Drawing for the job (mm, zero at the part's lowest x, y, z). Give positions to 0.01 mm unless a question says otherwise; leave off trailing zeros. Write each loop counter-clockwise with the first axis right and the second up, starting at its lowest first coordinate (ties: lowest second). Pieces come first, ordered by that corner, then holes. Notation, with made-up numbers: M 26.25,20.5 L 56.25,20.5 A30 cw 56.25,44.5 Z; hole C 74.5,67.5 d8. An arc over 180 degrees is marked long. Use CSV: the item, a comma, the result in double quotes. Start each with the question number.
1. Drill centre lines: line 1 along X through (y, z) = (14, 5); line 2 along X through (y, z) = (30.5, 7.25). Where is each one in solid material? Low to high. Write a range as from..to.
2. Drop flat-ended pins along their axis: pin 1 Ø1 at (y, z) = (12.5, 7) entering from +X; pin 2 Ø4 at (y, z) = (14.5, 7) entering from +X; pin 3 Ø3 at (x, y) = (68, 27.5) entering from -Z. Give the stop position or say it passes through.
3. Band-saw the part on A-A, the plane z = 7.75. List the corners of the cut face in (x, y) (3 decimals).
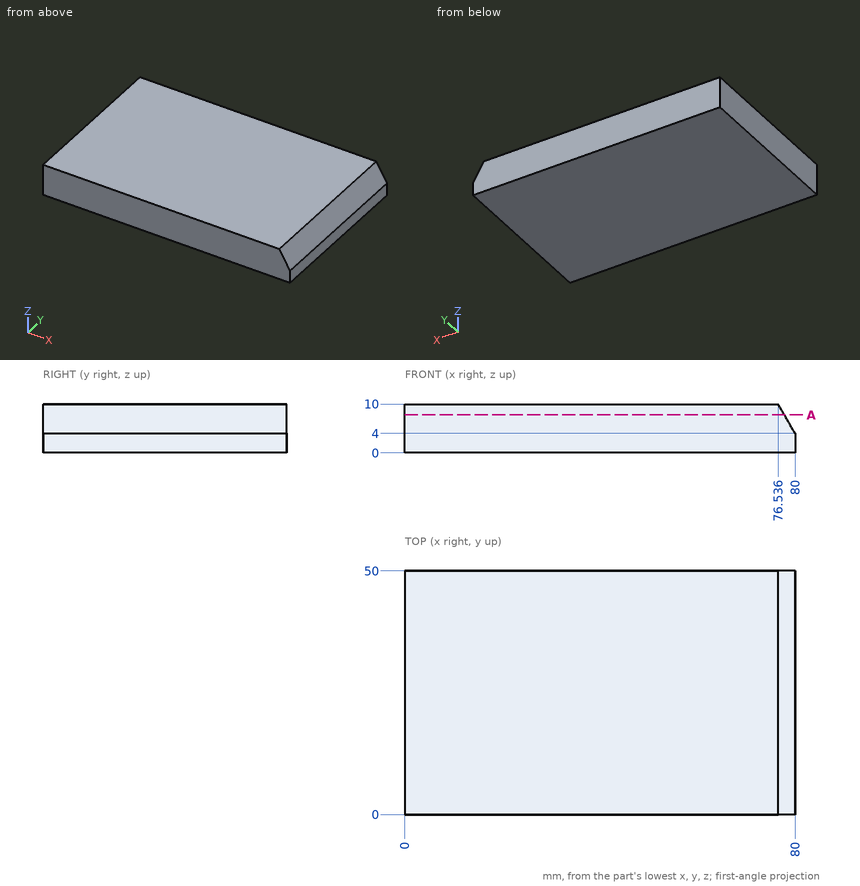
Output:
1,line 1,"x = 0..79.42"
1,line 2,"x = 0..78.12"
2,pin 1,"stops at x = 78.56"
2,pin 2,"stops at x = 79.42"
2,pin 3,"stops at z = 0"
3,outline,"M 0,0 L 77.835,0 L 77.835,50 L 0,50 Z"
